Part print with two shaded views. Sizes in mm from the minimum x, y, z corner. A direction names the side the tool comes from. Coordinates: 2 decimals unless noted, no trailing zeros. Loops run counter-clockwise (first coordinate to the right, second up) from the corner with the lowest first, then second, coordinate; pieces in that order, holes last.
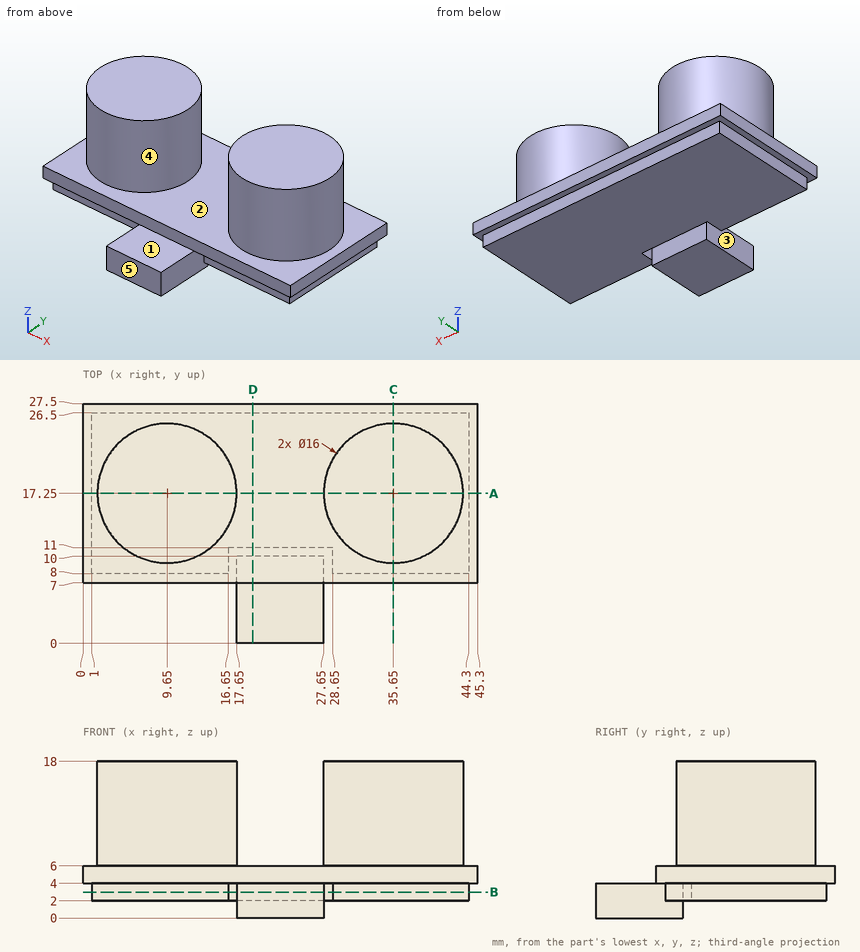
Q1. Flat gauge pins, fed straight in: P1, Ø0.6, axis at y = 19, z = 2.5, coming from the +X side; P2, Ø1.5, axis at y = 15, z = 10, coming from the -X side; P3, Ø5.5, axis at x = 25, y = 4, coming from the +Z side. Where does each tip first touch, or does it go through?
Answers:
P1: stops at x = 44.3
P2: stops at x = 1.79
P3: stops at z = 4
Q2. Slice it at C-C (x = 35.65). List the corners of the cut face in (y, z).
Answers:
outline: (7, 4) - (8, 4) - (8, 2) - (26.5, 2) - (26.5, 4) - (27.5, 4) - (27.5, 6) - (25.25, 6) - (25.25, 18) - (9.25, 18) - (9.25, 6) - (7, 6) - close
Q3. Slice it at D-D (x = 19.5). List the corners of the cut face in (y, z).
Answers:
outline: (0, 0) - (10, 0) - (10, 4) - (11, 4) - (11, 2) - (26.5, 2) - (26.5, 4) - (27.5, 4) - (27.5, 6) - (7, 6) - (7, 4) - (0, 4) - close
Q4. Which spindle directions (+Z, -Z, +X, -X, +Y, -Y) get a long thin tool onto all of the face, cutting with end or side? Do the marked faces 3, 4 and 5. Say none if no direction does.
Answers:
face 3: -Z, -Y
face 4: +Z
face 5: +Z, -Z, +X, -X, -Y
Q5. Mould opens along X. For the marked faces 1 and 2 say: +X half, -X half, draft (parallel to the pull), parting line (faces both ways), or undercut.
Answers:
face 1: draft
face 2: undercut
Q6. Slice it at B-B (z = 3). List the corners of the cut face in (x, y).
Answers:
outline: (1, 8) - (16.65, 8) - (16.65, 11) - (28.65, 11) - (28.65, 8) - (44.3, 8) - (44.3, 26.5) - (1, 26.5) - close; (17.65, 0) - (27.65, 0) - (27.65, 10) - (17.65, 10) - close
Q7. Drill centre lines: line 1 (Z direction, x = 31, y = 7.25); line 2 (Z direction, x = 40.5, y = 23.25); line 3 (X direction, y = 8.75, z = 1.5). Where is each one in solid material? Low to high.
Answers:
line 1: z = 4 to 6
line 2: z = 2 to 18
line 3: x = 17.65 to 27.65
Q8. Slice it at A-A (y = 17.25). List the corners of the cut face in (x, z), and give its area (3 significant figures).
Answers:
outline: (0, 4) - (1, 4) - (1, 2) - (44.3, 2) - (44.3, 4) - (45.3, 4) - (45.3, 6) - (43.65, 6) - (43.65, 18) - (27.65, 18) - (27.65, 6) - (17.65, 6) - (17.65, 18) - (1.65, 18) - (1.65, 6) - (0, 6) - close
area: 561 mm2
